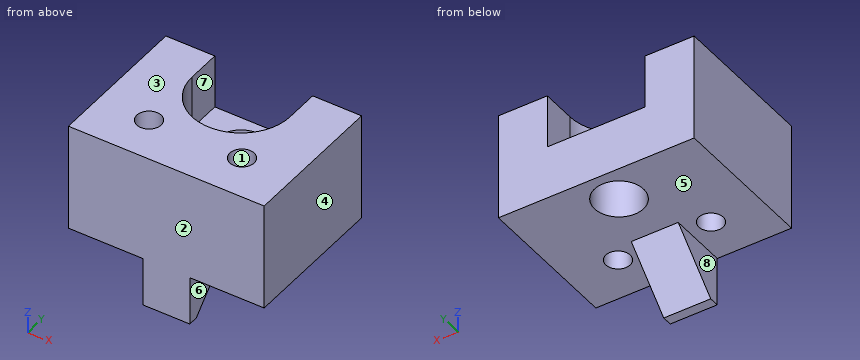
```python
from build123d import *

# Parameters (mm, degrees)
SKETCH1_W           = 20
SKETCH1_H           = 15
SKETCH1_R           = 2.5
SKETCH1_R_2         = 1.25
BOSS_EXTRUDE1_DEPTH = 11
CUT_EXTRUDE1_DEPTH  = 5.5
SKETCH3_W           = 4.8
SKETCH3_H           = 6
BOSS_EXTRUDE2_DEPTH = 5
CHAMFER1_SIZE       = 5


with BuildPart() as part:
    # Sketch1 → Boss-Extrude1 (new body)
    with BuildSketch(Plane.XY):
        with Locations((10, 7.5)):
            Rectangle(SKETCH1_W, SKETCH1_H)
        with Locations((10, 11.5)):
            Circle(SKETCH1_R, mode=Mode.SUBTRACT)
        with Locations((5.25, 4.5)):
            Circle(SKETCH1_R_2, mode=Mode.SUBTRACT)
        with Locations((14.75, 4.5)):
            Circle(SKETCH1_R_2, mode=Mode.SUBTRACT)
    extrude(amount=BOSS_EXTRUDE1_DEPTH)

    # Sketch2 → Cut-Extrude1 (cut)
    with BuildSketch(Plane.XY.offset(11)):
        with BuildLine():
            Line((15, 11.5), (15, 15))
            Line((15, 15), (5, 15))
            Line((5, 15), (5, 11.5))
            ThreePointArc((5, 11.5), (10, 6.5), (15, 11.5))
        make_face()
    extrude(amount=-CUT_EXTRUDE1_DEPTH, mode=Mode.SUBTRACT)

    # Sketch3 → Boss-Extrude2 (add)
    with BuildSketch(Plane(origin=(0, 0, 0), x_dir=(-1, 0, 0), z_dir=(0, 0, -1))):
        with Locations((-10, 3)):
            Rectangle(SKETCH3_W, SKETCH3_H)
    extrude(amount=BOSS_EXTRUDE2_DEPTH)

    # Chamfer1
    chamfer1_edges = [part.edges().sort_by_distance(p)[0] for p in [
        (10, 6, -5),
    ]]
    chamfer(chamfer1_edges, length=CHAMFER1_SIZE - 0.0001)  # a hair under: the kernel refuses the full size


solid = part.part
```
Read the model definition and answer for the solid it produces. Units are mm, in the model's axes. Face numbers are marked on the shaded views. A direction names the side the tool comes from. Give positions to 0.01 mm unless a question says otherwise; leave off trailing zeros. Write each loop counter-clockwise with the first axis right and the second up, starting at its lowest first coordinate (ties: lowest second). Pieces come first, ordered by that corner, then holes. Notation, with made-up numbers: M 11.25,-11 L 40.25,-11 A16 ccw 40.25,1 Z; hole C -6.5,-32.5 d1. An arc over 180 degrees is marked long. Put each result on its own line as item: value. Start each with the question number.
1. Each of these flat-tipped pins is pushed along its axis until it touches: pin 1 Ø1.5 at (x, z) = (10.5, -3) entering from +Y; pin 2 Ø6 at (x, y) = (10, 11.5) entering from -Z; pin 3 Ø4 at (x, y) = (14.75, 4.5) entering from +Z; pin 4 Ø1.5 at (y, z) = (4, -2) entering from -X. Where does it stop, or does it pass through?
2. Consider line 1 along Y through (x, z) = (14.75, 3); line 2 along Y through (x, z) = (10, 1.6); line 3 along X through (y, z) = (5.25, 4.75). Determine where each line is inside the solid, lowest interval first.
3. The part is cut by section C-C, the plane y = 4.5. Give the vertices of the cut face in (x, z), and give its area (3 significant figures).
4. The part is cut by section D-D, the plane y = 11.25. Give the vertices of the cut face in (x, z).
5. Which of the six approach directions +Z, -Z, +X, -X, +Y, -Y give full straight-line access (tool end or side, diameter ignored) to the marked faces 4, 5, 6, 7 and 8?
6. The part is cut by section B-B, the plane z = 2.5. Give the vertices of the cut face in (x, y), and give its area (3 significant figures).
7. For a pull along Y with two mould halves and no side action, classify the marked faces 1, 2 and 3 as released by +Y, released by -Y, zero draft, split by the parting line, or undercut.
Final values:
1. pin 1: stops at y = 3.75
1. pin 2: stops at z = 0
1. pin 3: stops at z = 11
1. pin 4: stops at x = 7.6
2. line 1: y = 0 to 3.25, 5.75 to 15
2. line 2: y = 0 to 9, 14 to 15
2. line 3: x = 0 to 4.25, 6.25 to 13.75, 15.75 to 20
3. outline: M 0,0 L 4,0 L 4,11 L 0,11 Z; M 6.5,0 L 7.6,0 L 7.6,-1.5 L 12.4,-1.5 L 12.4,0 L 13.5,0 L 13.5,11 L 6.5,11 Z; M 16,0 L 20,0 L 20,11 L 16,11 Z
3. area: 172 mm²
4. outline: M 0,0 L 7.51,0 L 7.51,5.5 L 5.01,5.5 L 5.01,11 L 0,11 Z; M 12.49,0 L 20,0 L 20,11 L 14.99,11 L 14.99,5.5 L 12.49,5.5 Z
5. face 4: +Z, -Z, +X, +Y, -Y
5. face 5: -Z, +Y
5. face 6: -Z, +X, +Y, -Y
5. face 7: +Z, +Y
5. face 8: -Z, -X, +Y, -Y
6. outline: M 0,0 L 20,0 L 20,15 L 0,15 Z; hole C 5.25,4.5 d2.5; hole C 10,11.5 d5; hole C 14.75,4.5 d2.5
6. area: 271 mm²
7. face 1: undercut
7. face 2: released by -Y
7. face 3: zero draft
